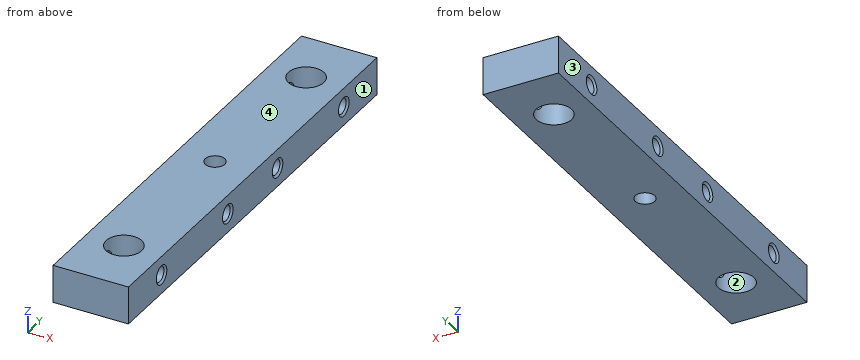
```python
from build123d import *

# Parameters (mm, degrees)
CROQUIS1_W                         = 25.4
CROQUIS1_H                         = 150
CROQUIS1_R                         = 6
SALIENTE_EXTRUIR1_DEPTH            = 6.35
TALADRO_ROSCADO_1_4_201_AT_2_COUNT = 2
TALADRO_ROSCADO_1_4_201_AT_2_PITCH = 30
TALADRO_ROSCADO_1_4_202_AT_2_COUNT = 2
TALADRO_ROSCADO_1_4_202_AT_2_PITCH = 110
TALADRO_DE_MARGEN_PARA_1_D         = 6.6


with BuildPart() as part:
    # Croquis1 → Saliente-Extruir1 (new, symmetric)
    with BuildSketch(Plane.XY):
        Rectangle(CROQUIS1_W, CROQUIS1_H)
        with Locations((0, 55)):
            Circle(CROQUIS1_R, mode=Mode.SUBTRACT)
        with Locations(Location((0, -55, 0), (0, 0, 180))):
            Circle(CROQUIS1_R, mode=Mode.SUBTRACT)
    extrude(amount=SALIENTE_EXTRUIR1_DEPTH, both=True)

    # Croquis3 → Taladro roscado 1/4-201 (revolve, cut)
    with BuildSketch(Plane(origin=(-12.7, -15, 0), x_dir=(0, 0, 1), z_dir=(0, 1, 0))):
        Polygon((0, 0), (0, 25.4), (3.1877, 25.4), (2.5527, 24.765), (2.5527, 0.635), (3.1877, 0), align=None)
    taladro_roscado_1_4_201 = revolve(axis=Axis((-19.05, -15, 0), (1, 0, 0)), mode=Mode.SUBTRACT)

    # Taladro roscado 1/4-201 at 2: Taladro roscado 1/4-201 ×2
    with Locations(*[(0, i * TALADRO_ROSCADO_1_4_201_AT_2_PITCH, 0) for i in range(1, TALADRO_ROSCADO_1_4_201_AT_2_COUNT)]):
        add(taladro_roscado_1_4_201, mode=Mode.SUBTRACT)

    # Croquis7 → Taladro roscado 1/4-202 (revolve, cut)
    with BuildSketch(Plane(origin=(-12.7, 55, 0), x_dir=(0, 0, 1), z_dir=(0, 1, 0))):
        Polygon((0, 0), (0, 25.4), (3.1877, 25.4), (2.5527, 24.765), (2.5527, 0.635), (3.1877, 0), align=None)
    taladro_roscado_1_4_202 = revolve(axis=Axis((-19.05, 55, 0), (1, 0, 0)), mode=Mode.SUBTRACT)

    # Taladro roscado 1/4-202 at 2: Taladro roscado 1/4-202 ×2
    with Locations(*[(0, -i * TALADRO_ROSCADO_1_4_202_AT_2_PITCH, 0) for i in range(1, TALADRO_ROSCADO_1_4_202_AT_2_COUNT)]):
        add(taladro_roscado_1_4_202, mode=Mode.SUBTRACT)

    # Taladro de margen para 1 (through all)
    with Locations(Plane.XY.offset(6.35)):
        with Locations((0, 0)):
            Hole(TALADRO_DE_MARGEN_PARA_1_D / 2)


solid = part.part
```
The model under review builds one solid part; all positions refer to its coordinate system, in mm. Face numbers are marked on the shaded views. Coordinates: 2 decimals unless noted, no trailing zeros. Write each loop counter-clockwise with the first axis right and the second up, starting at its lowest first coordinate (ties: lowest second). Pieces come first, ordered by that corner, then holes.
1) We need section A-A on y = 0. State the section outline as (x, z) points, then the cut area to 3 significant figures.
2) We need section C-C on x = 10.5. State the section outline as (y, z) points.
3) To check wall thickness, follow probe 1 along Y at (x, z) = (10.25, 0); probe 2 along X at (y, z) = (-60, 4.5); probe 3 along Y at (x, z) = (-5, -0.25). State the ranges of each line that lie inside material, in increasing order.
4) The part is to be moulded in two halves that separate along X. For the marked faces 1, 2, 3 and 4, say which applies: pulls with the +X half, pulls with the -X half, needs draft (parallel to the pull), parting line crosses it, or undercut.
5) We need section B-B on x = 0. State the section outline as (y, z) points.
6) Clearance check with a flat-ended pin moving along its axis: pin 1 Ø6.5 at (y, z) = (55, 0) entering from +X. State where the tip first meets the part, or that it passes through.
7) We need section D-D on z = 4.5. State the section outline as (x, y) points.
Answer list:
1. outline: (-12.7, -6.35) - (-3.3, -6.35) - (-3.3, 6.35) - (-12.7, 6.35) - close; (3.3, -6.35) - (12.7, -6.35) - (12.7, 6.35) - (3.3, 6.35) - close
1. area: 239 mm2
2. outline: (-75, -6.35) - (75, -6.35) - (75, 6.35) - (-75, 6.35) - close; hole circle Ø5.11 at (-55, 0); hole circle Ø5.11 at (-15, 0); hole circle Ø5.11 at (15, 0); hole circle Ø5.11 at (55, 0)
3. probe 1: y = -75 to -57.55, -52.45 to -17.55, -12.45 to 12.45, 17.55 to 52.45, 57.55 to 75
3. probe 2: x = -12.7 to -3.32, 3.32 to 12.7
3. probe 3: y = -75 to -58.32, -51.68 to -17.54, -12.46 to 12.46, 17.54 to 51.68, 58.32 to 75
4. face 1: pulls with the +X half
4. face 2: undercut
4. face 3: pulls with the -X half
4. face 4: needs draft
5. outline: (-75, -6.35) - (-61, -6.35) - (-61, 6.35) - (-75, 6.35) - close; (-49, -6.35) - (-3.3, -6.35) - (-3.3, 6.35) - (-49, 6.35) - close; (3.3, -6.35) - (49, -6.35) - (49, 6.35) - (3.3, 6.35) - close; (61, -6.35) - (75, -6.35) - (75, 6.35) - (61, 6.35) - close; hole circle Ø5.11 at (-15, 0); hole circle Ø5.11 at (15, 0)
6. pin 1: stops at x = 12.7
7. outline: (-12.7, -75) - (12.7, -75) - (12.7, 75) - (-12.7, 75) - close; hole circle Ø12 at (0, -55); hole circle Ø12 at (0, 55); hole circle Ø6.6 at (0, 0)
